```python
from build123d import *

# Parameters (mm, degrees)
F0_W      = 25
F0_H      = 24
F1_DEPTH  = 0.8
F2_W      = 8
F2_H      = 8
F3_DEPTH  = 3.2
F4_R      = 3.75
F5_DEPTH  = 1
F6_R      = 3
F7_DEPTH  = 1
F9_D      = 2
F10_W     = 8
F10_H     = 5
F11_DEPTH = 1.6
F13_DEPTH = 2.6
F14_W     = 16
F14_H     = 0.15
F15_DEPTH = 25


with BuildPart() as f1:
    # F0 (on Top) → F1 (new body)
    with BuildSketch(Plane.XY):
        with Locations((0, 2.5)):
            Rectangle(F0_W, F0_H)
    extrude(amount=-F1_DEPTH)

    # F2 (on face) → F3 (join)
    with BuildSketch(Plane.XY):
        Rectangle(F2_W, F2_H)
    extrude(amount=F3_DEPTH)

    # F4 (on face) → F5 (join)
    with BuildSketch(Plane.XY.offset(3.2)):
        Circle(F4_R)
    extrude(amount=F5_DEPTH)

    # F6 (on face) → F7 (join)
    with BuildSketch(Plane.XY.offset(4.2)):
        Circle(F6_R)
    extrude(amount=F7_DEPTH)

    # F9 (through all)
    with Locations(Plane.XY):
        with Locations((-10.5, 12.5), (10.5, 12.5), (10.5, 0), (-10.5, 0)):
            Hole(F9_D / 2)

    # F10 (on face) → F11 (join)
    with BuildSketch(Plane.XY):
        with Locations((0, 10.5)):
            Rectangle(F10_W, F10_H)
    extrude(amount=F11_DEPTH)

    # F12 (on face) → F13 (join)
    with BuildSketch(Plane(origin=(0, 0, -0.8), x_dir=(1, 0, 0), z_dir=(0, 0, -1))):
        Polygon((11.5, 9.5), (-11.5, 9.5), (-11.5, 8.6), (-10.1, 8.6), (-10.1, 4), (10.1, 4), (10.1, 8.6), (11.5, 8.6), align=None)
    extrude(amount=F13_DEPTH)

    # F14 (on face) → F15 (join)
    with BuildSketch(Plane.XZ.offset(9.5)):
        with Locations((0, -2.075)):
            Rectangle(F14_W, F14_H)
    extrude(amount=F15_DEPTH)


solid = f1.part
```
Input: part model. Units: mm. Frame: model coordinates. A direction names the side the tool comes from. Coordinates: 2 decimals unless noted, no trailing zeros. Write each loop counter-clockwise with the first axis right and the second up, starting at its lowest first coordinate (ties: lowest second). Pieces come first, ordered by that corner, then holes.
1) Pin query (flat end, axial travel): pin 1 Ø2 at (x, y) = (8.5, -25) entering from -Z; pin 2 Ø0.8 at (y, z) = (11, 0.5) entering from +X; pin 3 Ø0.7 at (x, z) = (-10.5, -2.5) entering from +Y. Return the tip coordinate at first contact, or that it passes through.
2) Section A-A on y = 0. Output: boundary loops of the cut face in (x, z).
3) Section B-B on x = 1. Output: boundary loops of the cut face in (y, z).
4) Section D-D on y = -13. Output: boundary loops of the cut face in (x, z), and give its area (3 significant figures).
5) Section C-C on z = 2.5. Output: boundary loops of the cut face in (x, y), and give its area (3 significant figures).
6) Set-up query: faces 4 (the flat face through (0, 8, 1)), 5 (the flat face through (10.1, -6, -2)), 6 (the flat face through (-4, 10, 1)), 7 (the flat face through (-3, 3, 3.2)), 8 (the flat face through (0, -4, -2)). Return all of +Z, -Z, +X, -X, +Y, -Y with unobstructed straight access to the full face (end or side cutting, diameter ignored); none if empty.
7) Mould query, pull axis X, two halves, no side actions, for faces 1 (the flat face through (0, 5, 0)), 2 (the flat face through (4, 10, 1)), 3 (the cylindrical face through (-9.7, -0.6, -0.4)). Classes: pulls with the +X half, pulls with the -X half, needs draft (parallel to the pull), parting line crosses it, or undercut.
8) Material intervals for line 1 along Y through (x, z) = (10.5, -0.35); line 2 along Z through (x, y) = (2.25, 10.5); line 3 along Z through (x, y) = (3.5, -2.5), sorted ascending.
Check result:
1. pin 1: stops at z = -2.15
1. pin 2: stops at x = 4
1. pin 3: stops at y = -8.6
2. outline: (-12.5, -0.8) - (-11.5, -0.8) - (-11.5, 0) - (-12.5, 0) - close; (-9.5, -0.8) - (9.5, -0.8) - (9.5, 0) - (4, 0) - (4, 3.2) - (3.75, 3.2) - (3.75, 4.2) - (3, 4.2) - (3, 5.2) - (-3, 5.2) - (-3, 4.2) - (-3.75, 4.2) - (-3.75, 3.2) - (-4, 3.2) - (-4, 0) - (-9.5, 0) - close; (11.5, -0.8) - (12.5, -0.8) - (12.5, 0) - (11.5, 0) - close
3. outline: (-34.5, -2.15) - (-9.5, -2.15) - (-9.5, -3.4) - (-4, -3.4) - (-4, -0.8) - (14.5, -0.8) - (14.5, 0) - (13, 0) - (13, 1.6) - (8, 1.6) - (8, 0) - (4, 0) - (4, 3.2) - (3.61, 3.2) - (3.61, 4.2) - (2.83, 4.2) - (2.83, 5.2) - (-2.83, 5.2) - (-2.83, 4.2) - (-3.61, 4.2) - (-3.61, 3.2) - (-4, 3.2) - (-4, 0) - (-9.5, 0) - (-9.5, -2) - (-34.5, -2) - close
4. outline: (-8, -2.15) - (8, -2.15) - (8, -2) - (-8, -2) - close
4. area: 2.40 mm2
5. outline: (-4, -4) - (4, -4) - (4, 4) - (-4, 4) - close
5. area: 64.0 mm2
6. face 4: +Z, +X, -X
6. face 5: -Z, +X, +Y
6. face 6: +Z, -X, +Y, -Y
6. face 7: +Z
6. face 8: -Z, +X, -X, +Y
7. face 1: needs draft
7. face 2: pulls with the +X half
7. face 3: undercut
8. line 1: y = -9.5 to -1, 1 to 11.5, 13.5 to 14.5
8. line 2: z = -0.8 to 1.6
8. line 3: z = -0.8 to 3.2
